Autodesk Inventor part; units mm, degrees
ref_plane "YZ Plane" through (0, 0, 0) normal (1, 0, 0) x (0, 1, 0)
ref_plane "XZ Plane" through (0, 0, 0) normal (0, 1, 0) x (-1, 0, 0)
ref_plane "XY Plane" through (0, 0, 0) normal (0, 0, 1) x (1, 0, 0)
sketch "Sketch5" plane through (0, 0, 0) normal (0, 0, 1) x (1, 0, 0)
  line L0 (-42.5, 97.5) -> (42.5, 97.5)
  line L1 (42.5, 97.5) -> (42.5, -97.5)
  line L2 (42.5, -97.5) -> (-42.5, -97.5)
  line L3 (-42.5, -97.5) -> (-42.5, 97.5)
  point P0 (0, 0)
  point P1 (0, 97.5)
  point P2 (42.5, 0)
  point P3 (-42.5, 0)
  dimension "d8" = 195
  dimension "d9" = 85
extrude "Extrusion5" add sketch "Sketch5" along normal mid plane 15
sketch "Sketch6" plane through (0, 0, 7.5) normal (0, 0, 1) x (1, 0, 0)
  line L0 (42.5, -97.5) -> (16.5, -97.5)
  line L1 (16.5, -97.5) -> (16.5, -9.5)
  line L2 (16.5, -9.5) -> (42.5, -9.5)
  line L3 (42.5, -9.5) -> (42.5, -97.5)
  point P0 (0, 0)
  dimension "d12" = 88
  dimension "d13" = 26
extrude "Extrusion6" cut sketch "Sketch6" against normal blind 15
sketch "Sketch7" plane through (0, 0, 7.5) normal (0, 0, 1) x (1, 0, 0)
  line L0 (42.5, 97.5) -> (-42.5, 97.5)
  line L1 (-42.5, 97.5) -> (-42.5, -97.5)
  line L2 (-42.5, -97.5) -> (16.5, -97.5)
  circle A0 centre (31.5, 83.75) radius 4.25
  circle A1 centre (31.5, 43.75) radius 4.25
  circle A2 centre (31.5, 3.75) radius 4.25
  circle A3 centre (-33.5, -82.5) radius 4.25
  circle A4 centre (6.5, -82.5) radius 4.25
  line L3 (16.5, -97.5) -> (16.5, -9.5)
  line L4 (42.5, -9.5) -> (42.5, 97.5)
  point P0 (0, 0)
  dimension "d17" = 74
  dimension "d18" = 8.5
  dimension "d19" = 40
  dimension "d20" = 40
  dimension "d21" = 13.75
  dimension "d22" = 40
  dimension "d23" = 15
  dimension "d66" = 10
  dimension "d68" = 11
hole "Hole1" at (31.5, 83.75, 7.5) at (31.5, 43.75, 7.5) at (31.5, 3.75, 7.5) at (6.5, -82.5, 7.5) at (-33.5, -82.5, 7.5) direction (0, 0, -1) diameter 8.5 end through all counterbore diameter 14 counterbore depth 9
sketch "Sketch8" plane through (0, 0, 7.5) normal (0, 0, 1) x (1, 0, 0)
  line L0 (42.5, 97.5) -> (-42.5, 97.5)
  line L1 (-42.5, 97.5) -> (-42.5, -97.5)
  line L2 (-42.5, -97.5) -> (16.5, -97.5)
  circle A0 centre (-28.5, 85) radius 4
  circle A1 centre (1.5, 85) radius 4
  circle A2 centre (-28.5, 55) radius 4
  circle A3 centre (1.5, 55) radius 4
  circle A4 centre (-28.5, 30) radius 4
  circle A5 centre (-28.5, 0) radius 4
  circle A6 centre (1.5, 30) radius 4
  circle A7 centre (1.5, 0) radius 4
  circle A8 centre (-28.5, -55) radius 4
  circle A9 centre (1.5, -55) radius 4
  line L3 (-57.3365, -67.5) -> (43.3911, -67.5)
  line L4 (-57.3365, -12.5) -> (43.3911, -12.5)
  line L5 (-57.3365, 42.5) -> (43.3911, 42.5)
  circle A10 centre (-28.5, -25) radius 4
  circle A11 centre (1.5, -25) radius 4
  point P0 (0, 0)
  dimension "d33" = 8
  dimension "d34" = 30
  dimension "d36" = 55
  dimension "d37" = 55
  dimension "d38" = 30
  dimension "d39" = 55
  dimension "d40" = 12.5
  dimension "d41" = 12.5
  dimension "d42" = 30
  dimension "d43" = 12.5
  dimension "d44" = 30
  dimension "d45" = 30
  dimension "d46" = 14
hole "Hole2" at (-28.5, 85, 7.5) at (1.5, 85, 7.5) at (1.5, 55, 7.5) at (-28.5, 55, 7.5) at (-28.5, 30, 7.5) at (1.5, 30, 7.5) at (1.5, 0, 7.5) at (-28.5, 0, 7.5) at (-28.5, -25, 7.5) at (1.5, -25, 7.5) at (1.5, -55, 7.5) at (-28.5, -55, 7.5) direction (0, 0, -1) diameter 6.647 end through all
sketch "Sketch9" plane through (-42.5, -97.5, 7.5) normal (-1, 0, 0) x (0, 0, 1)
  line L0 (-15, 195) -> (0, 195)
  circle A0 centre (-7.5, 167.5) radius 3
  circle A1 centre (-7.5, 112.5) radius 3
  circle A2 centre (-7.5, 57.5) radius 3
  line L1 (0, 0) -> (-15, 0)
  point P0 (-7.5, 97.5)
  point P1 (-7.5, 97.5)
  dimension "d55" = 55
  dimension "d56" = 55
  dimension "d57" = 6
  dimension "d65" = 57.5
hole "Hole3" at (-42.5, -40, 0) at (-42.5, 15, 0) at (-42.5, 70, 0) direction (1, 0, 0) diameter 4.917 depth 15 tip angle 118
equation "\"d20\" = d19"
properties part number "BC-10014" material "Alumínio 7075"
Design review of the part built by this model. Coordinates are the model's own, in mm. A direction names the side the tool comes from. Give positions to 0.01 mm unless a question says otherwise; leave off trailing zeros. Write each loop counter-clockwise with the first axis right and the second up, starting at its lowest first coordinate (ties: lowest second). Pieces come first, ordered by that corner, then holes. Notation, with made-up numbers: (85.25, 45) - (137.25, 45) arc R18 cw to (137.25, 50) - close; hole circle Ø2 at (49.25, 26.5). An arc over 180 degrees is marked (long way). Return JSON: item names as keys, results as strings. Group by question number.
(1) Mouldability with a two-part tool opening along Z and no side actions: class faces 4 (the cylindrical face through (-34.89, 72.4, -0.53)), 5 (the cylindrical face through (1.35, -51.68, -0.11)), 6 (the flat face through (35, 1, -1.5)) as +Z half, -Z half, draft (parallel to the pull), parting line (faces both ways), or undercut.
(2) Insertion check: pin 1 (10 mm diameter, centred on x = 6.5, y = -82.5, fed in from +Z); pin 2 (8.5 mm diameter, centred on x = 1.5, y = -55, fed in from -Z). Each pin has a flat end and moves straight along its axis. Give the tip position at first contact, or say it passes through.
(3) To check wall thickness, follow probe 1 along Y at (x, z) = (31.5, 5.25); probe 2 along Y at (x, z) = (31.5, -4.8); probe 3 along X at (y, z) = (30, 0). State the ranges of each line that lie inside material, in increasing order.
(4) We need section C-C, the plane y = 54.5. Give the boundary of the cut face in (x, z).
(5) Machinability: for faces 1 (the cylindrical face through (-34.895, 12.562, -0.32)), 2 (the flat face through (35, 41, -1.5)), 3 (the cylindrical face through (-30.746, 32.45, -0.105)), which of the approach directions +Z, -Z, +X, -X, +Y, -Y give a long, thin tool a straight path to every point of the face, cutting with its end or side? Answer none if there is none.
(6) We need section A-A, the plane z = 5.75. Give the number of separate pieces and of enclosed holes in the cut face, then the cut area to 3 significant figures.
(7) We need section B-B, the plane y = 83.75. Give the boundary of the cut face in (x, z), then the cut area to 3 significant figures.
Reported:
{
 "1": {"face 4": "undercut", "face 5": "draft", "face 6": "+Z half"},
 "2": {"pin 1": "stops at z = -1.5", "pin 2": "stops at z = -7.5"},
 "3": {"probe 1": "y = -9.5 to -3.25, 10.75 to 36.75, 50.75 to 76.75, 90.75 to 97.5", "probe 2": "y = -9.5 to -0.5, 8 to 39.5, 48 to 79.5, 88 to 97.5", "probe 3": "x = -42.5 to -31.82, -25.18 to -1.82, 4.82 to 42.5"},
 "4": {"outline": "(-42.5, -7.5) - (-31.79, -7.5) - (-31.79, 7.5) - (-42.5, 7.5) - close; (-25.21, -7.5) - (-1.79, -7.5) - (-1.79, 7.5) - (-25.21, 7.5) - close; (4.79, -7.5) - (42.5, -7.5) - (42.5, 7.5) - (4.79, 7.5) - close"},
 "5": {"face 1": "-X", "face 2": "+Z", "face 3": "+Z, -Z"},
 "6": {"separate pieces": "1", "enclosed holes": "17", "area": "13,100 mm2"},
 "7": {"outline": "(-42.5, -7.5) - (-31.58, -7.5) - (-31.58, 7.5) - (-42.5, 7.5) - close; (-25.42, -7.5) - (-1.58, -7.5) - (-1.58, 7.5) - (-25.42, 7.5) - close; (4.58, -7.5) - (27.25, -7.5) - (27.25, -1.5) - (24.5, -1.5) - (24.5, 7.5) - (4.58, 7.5) - close; (35.75, -7.5) - (42.5, -7.5) - (42.5, 7.5) - (38.5, 7.5) - (38.5, -1.5) - (35.75, -1.5) - close", "area": "913 mm2"}
}
